from build123d import *

# Parameters (mm, degrees)
SKETCH1_R           = 1.27
BOSS_EXTRUDE1_DEPTH = 3.175
FILLET3_R           = 2.54


with BuildPart() as part:
    # Sketch1 → Boss-Extrude1 (new body)
    with BuildSketch(Plane(origin=(0, 0, 0), x_dir=(0, 0, -1), z_dir=(1, 0, 0))):
        Polygon((0.846258814, 2.623762197), (9.840144814, 2.623762197), (9.840144814, 25.789873149), (0.846258814, 25.789873149), (-14.571831472, 25.789873149), (-14.571831472, 14.187329911), (-6.773741186, 2.623762197), align=None)
        with Locations((5.343201814, 21.777648197)):
            Circle(SKETCH1_R, mode=Mode.SUBTRACT)
        with Locations((5.343201814, 11.617648197)):
            Circle(SKETCH1_R, mode=Mode.SUBTRACT)
        with Locations((-8.770559864, 19.98860153)):
            Circle(SKETCH1_R, mode=Mode.SUBTRACT)
    extrude(amount=BOSS_EXTRUDE1_DEPTH)

    # Fillet3
    fillet3_edges = [part.edges().sort_by_distance(p)[0] for p in [
        (1.5875, 25.789873149, -9.840144814),
    ]]
    fillet(fillet3_edges, radius=FILLET3_R)


solid = part.part
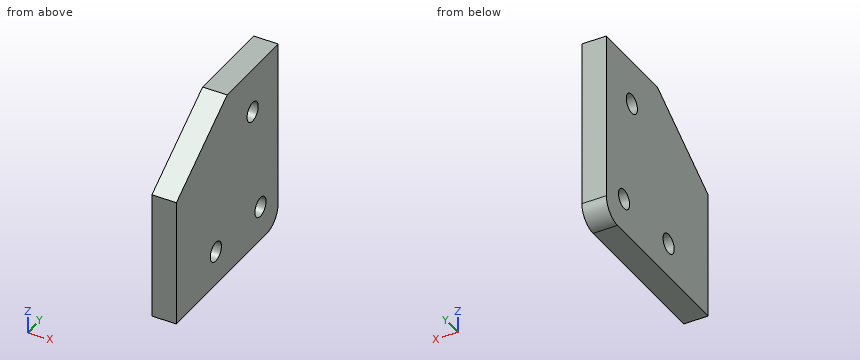
Model file for the job. Use its own axes, mm. Round coordinates to 2 decimals unless told otherwise and drop trailing zeros. Order: outer loops, then holes, each group sorted by start corner. A loop starts at its lowest first (then second) coordinate and runs counter-clockwise, first axis right, second up. Notation, with made-up numbers: M 55.5,60.5 L 68.5,60.5 A36 cw 68.5,98.5 Z; hole C 88,67 d2. An arc over 180 degrees is marked long. Write each question's results on one line, items separated by ' | '. Start each with the question number.
(1) Saw through at C-C, the plane z = 8.5. Give the cut face in (x, y) (3 decimals).
(2) Saw through at B-B, the plane x = 2.55. Give the cut face in (y, z), then the cut area to 3 significant figures.
(3) Saw through at D-D, the plane y = 5.5. Give the cut face in (x, z) (3 decimals), then the cut area to 3 significant figures.
(4) Probe probe 1 along Y at (x, z) = (2.15, -5.75); probe 2 along Z at (x, y) = (1.7, 19.25); probe 3 along Z at (x, y) = (0.5, 21.5). List the from-to ranges inside material, lowest first. Write a range as from..to.
(5) Saw through at A-A, the plane z = -5.5. Give the cut face in (x, y) (3 decimals), then the cut area to 3 significant figures.
Established:
1) outline: M 0,5.184 L 3.175,5.184 L 3.175,18.748 L 0,18.748 Z; M 0,21.229 L 3.175,21.229 L 3.175,25.79 L 0,25.79 Z
2) outline: M 2.62,-9.84 L 23.25,-9.84 A2.54 ccw 25.79,-7.3 L 25.79,14.57 L 14.19,14.57 L 2.62,6.77 Z; hole C 11.62,-5.34 d2.54; hole C 19.99,8.77 d2.54; hole C 21.78,-5.34 d2.54 | area: 504 mm^2
3) outline: M 0,-9.84 L 3.175,-9.84 L 3.175,8.713 L 0,8.713 Z | area: 58.9 mm^2
4) probe 1: y = 2.62..10.41, 12.82..20.57, 22.98..25.79 | probe 2: z = -9.84..7.74, 9.8..14.57 | probe 3: z = -9.84..-6.58, -4.1..14.57
5) outline: M 0,2.624 L 3.175,2.624 L 3.175,10.357 L 0,10.357 Z; M 0,12.878 L 3.175,12.878 L 3.175,20.517 L 0,20.517 Z; M 0,23.038 L 3.175,23.038 L 3.175,25.79 L 0,25.79 Z | area: 57.5 mm^2
